Model file for the job. Use its own axes, mm. A direction names the side the tool comes from. Give positions to 0.01 mm unless a question says otherwise; leave off trailing zeros. Loops run counter-clockwise (first coordinate to the right, second up) from the corner with the lowest first, then second, coordinate; pieces in that order, holes last. Notation, with made-up numbers: M 85,32.5 L 108,32.5 A23 ccw 108,64.5 Z; hole C -1.75,62 d6. An arc over 180 degrees is marked long. Answer in a Markdown table with one row per item.
```python
from build123d import *

# Parameters (mm, degrees)
SKETCH1_R           = 2.1
BOSS_EXTRUDE1_DEPTH = 6.3


with BuildPart() as part:
    # Sketch1 → Boss-Extrude1 (new body)
    with BuildSketch(Plane.XY):
        Polygon((33.4, 0), (-33.4, 0), (-33.4, 3), (-32.25, 3), (-32.25, 5.45), (-33.4, 5.45), (-33.4, 8.45), (-36.6, 8.45), (-36.6, 5.45), (-37.75, 5.45), (-37.75, 3), (-36.6, 3), (-36.6, 0), (-43, 0), (-43, 16), (43, 16), (43, 0), (36.6, 0), (36.6, 3), (37.75, 3), (37.75, 5.45), (36.6, 5.45), (36.6, 8.45), (33.4, 8.45), (33.4, 5.45), (32.25, 5.45), (32.25, 3), (33.4, 3), align=None)
        with Locations((-25, 11)):
            Circle(SKETCH1_R, mode=Mode.SUBTRACT)
        with Locations(Location((25, 11, 0), (0, 0, 180))):
            Circle(SKETCH1_R, mode=Mode.SUBTRACT)
    extrude(amount=BOSS_EXTRUDE1_DEPTH)


solid = part.part
```
Q1. Drop flat-ended pins along their axis: pin 1 (4 mm diameter, centred on x = -25, y = 11, fed in from -Z) (3 decimals); pin 2 (1 mm diameter, centred on x = -35, z = 3, fed in from -Y). Give the stop position or say it passes through.
Reported:
| item | result |
|---|---|
| pin 1 | through |
| pin 2 | y = 8.45 |
Q2. 3-axis set-ups, long thin cutter, end or side, ignore diameter. For faces 1 (the face through (-43, 8, 3)), 2 (the face through (-36.6, 7, 3)), 3 (the face through (37.75, 4, 3)): which of +Z, -Z, +X, -X, +Y, -Y reach the whole face in a straight line?
Reported:
| item | result |
|---|---|
| face 1 | +Z, -Z, -X, +Y, -Y |
| face 2 | +Z, -Z, -Y |
| face 3 | +Z, -Z |
Q3. Saw through at C-C (z = 4.5). Give the number of separate pieces and of enclosed holes in the cut face, and give its area (3 significant figures).
Reported:
| item | result |
|---|---|
| separate pieces | 1 |
| enclosed holes | 2 |
| area | 1,280 mm² |
Q4. Saw through at D-D (y = 11). Give the cut face in (x, z).
Reported:
| item | result |
|---|---|
| outline | M -43,0 L -27.1,0 L -27.1,6.3 L -43,6.3 Z; M -22.9,0 L 22.9,0 L 22.9,6.3 L -22.9,6.3 Z; M 27.1,0 L 43,0 L 43,6.3 L 27.1,6.3 Z |
Q5. Saw through at B-B (y = 1.25). Give the cut face in (x, z).
Reported:
| item | result |
|---|---|
| outline | M -43,0 L -36.6,0 L -36.6,6.3 L -43,6.3 Z; M -33.4,0 L 33.4,0 L 33.4,6.3 L -33.4,6.3 Z; M 36.6,0 L 43,0 L 43,6.3 L 36.6,6.3 Z |
Q6. Saw through at A-A (x = -25). Give the cut face in (y, z).
Reported:
| item | result |
|---|---|
| outline | M 0,0 L 8.9,0 L 8.9,6.3 L 0,6.3 Z; M 13.1,0 L 16,0 L 16,6.3 L 13.1,6.3 Z |
Q7. Probe probe 1 along X at (y, z) = (4, 5.75); probe 2 along X at (y, z) = (8, 0.75); probe 3 along Y at (x, z) = (25, 3). List the from-to ranges inside material, lowest first.
Reported:
| item | result |
|---|---|
| probe 1 | -43 to -37.75, -32.25 to 32.25, 37.75 to 43 |
| probe 2 | -43 to -36.6, -33.4 to 33.4, 36.6 to 43 |
| probe 3 | 0 to 8.9, 13.1 to 16 |
Q8. Mould opens along Y. For faces 4 (the face through (32.25, 4, 3)), 5 (the face through (-37.75, 4, 3)), 6 (the face through (33.4, 7, 3)), 7 (the face through (-1, 16, 3)) say: released by +Y, released by -Y, zero draft, split by the parting line, or undercut.
Reported:
| item | result |
|---|---|
| face 4 | undercut |
| face 5 | undercut |
| face 6 | zero draft |
| face 7 | released by +Y |
